```python
from build123d import *

# Parameters (mm, degrees)
SKETCH2_W           = 30.4
SKETCH2_H           = 30.4
BOSS_EXTRUDE1_DEPTH = 6
FILLET1_R           = 5
FILLET2_R           = 1
CUT_EXTRUDE1_DEPTH  = 0.5
BOSS_EXTRUDE2_DEPTH = 6.6
CUT_EXTRUDE2_DEPTH  = 10.6
FILLET3_R           = 1
CUT_EXTRUDE3_REACH  = 32.4
SKETCH9_W           = 0.8
SKETCH9_H           = 5.55
BOSS_EXTRUDE5_DEPTH = 2.35
LPATTERN1_COUNT     = 5
LPATTERN1_PITCH     = 2.78
SKETCH10_W          = 11.92
SKETCH10_H          = 2.35
BOSS_EXTRUDE6_DEPTH = 1
BOSS_EXTRUDE7_DEPTH = 1.65
SKETCH12_R          = 3.5
SKETCH12_R_2        = 2.5
BOSS_EXTRUDE8_DEPTH = 3.99
BOSS_EXTRUDE9_DEPTH = 1.6


with BuildPart() as part:
    # Sketch2 → Boss-Extrude1 (new body)
    with BuildSketch(Plane.XZ.offset(1.6)):
        with Locations((0, -13.5)):
            Rectangle(SKETCH2_W, SKETCH2_H)
    extrude(amount=BOSS_EXTRUDE1_DEPTH)

    # Fillet1
    fillet1_edges = [part.edges().sort_by_distance(p)[0] for p in [
        (15.2, -4.6, -28.7),
        (-15.2, -4.6, -28.7),
        (-15.2, -4.6, 1.7),
        (15.2, -4.6, 1.7),
    ]]
    fillet(fillet1_edges, radius=FILLET1_R)

    # Fillet2
    fillet2_edges = [part.edges().sort_by_distance(p)[0] for p in [
        (0, -7.6, 1.7),
        (15.2, -7.6, -13.5),
        (-15.2, -7.6, -13.5),
        (0, -7.6, -28.7),
        (-13.735533906, -7.6, -27.235533906),
        (-13.735533906, -7.6, 0.235533906),
        (13.735533906, -7.6, -27.235533906),
        (13.735533906, -7.6, 0.235533906),
    ]]
    fillet(fillet2_edges, radius=FILLET2_R)

    # Sketch3 → Cut-Extrude1 (cut)
    with BuildSketch(Plane.XZ.offset(7.6)):
        with BuildLine():
            Line((10.2, -1.8), (-10.2, -1.8))
            ThreePointArc((-10.2, -1.8), (-11.260660172, -2.239339828), (-11.7, -3.3))
            Line((-11.7, -3.3), (-11.7, -23.7))
            ThreePointArc((-11.7, -23.7), (-11.260660172, -24.760660172), (-10.2, -25.2))
            Line((-10.2, -25.2), (10.2, -25.2))
            ThreePointArc((10.2, -25.2), (11.260660172, -24.760660172), (11.7, -23.7))
            Line((11.7, -23.7), (11.7, -3.3))
            ThreePointArc((11.7, -3.3), (11.260660172, -2.239339828), (10.2, -1.8))
        make_face()
    extrude(amount=-CUT_EXTRUDE1_DEPTH, mode=Mode.SUBTRACT)

    # Sketch4 → Boss-Extrude2 (add)
    with BuildSketch(Plane(origin=(0, -1.6, 0), x_dir=(1, 0, 0), z_dir=(0, 1, 0))):
        with BuildLine():
            Line((15.2, 23.7), (15.2, 3.3))
            ThreePointArc((15.2, 3.3), (13.735533906, -0.235533906), (10.2, -1.7))
            Line((10.2, -1.7), (-10.2, -1.7))
            ThreePointArc((-10.2, -1.7), (-13.735533906, -0.235533906), (-15.2, 3.3))
            Line((-15.2, 3.3), (-15.2, 23.7))
            ThreePointArc((-15.2, 23.7), (-13.735533906, 27.235533906), (-10.2, 28.7))
            Line((-10.2, 28.7), (10.2, 28.7))
            ThreePointArc((10.2, 28.7), (13.735533906, 27.235533906), (15.2, 23.7))
        make_face()
    extrude(amount=BOSS_EXTRUDE2_DEPTH)

    # Sketch5 → Cut-Extrude2 (cut)
    with BuildSketch(Plane(origin=(0, 5, 0), x_dir=(1, 0, 0), z_dir=(0, 1, 0))):
        with BuildLine():
            Line((10.2, 27.2), (-10.2, 27.2))
            ThreePointArc((-10.2, 27.2), (-12.674873734, 26.174873734), (-13.7, 23.7))
            Line((-13.7, 23.7), (-13.7, 3.3))
            ThreePointArc((-13.7, 3.3), (-12.674873734, 0.825126266), (-10.2, -0.2))
            Line((-10.2, -0.2), (10.2, -0.2))
            ThreePointArc((10.2, -0.2), (12.674873734, 0.825126266), (13.7, 3.3))
            Line((13.7, 3.3), (13.7, 23.7))
            ThreePointArc((13.7, 23.7), (12.674873734, 26.174873734), (10.2, 27.2))
        make_face()
    extrude(amount=-CUT_EXTRUDE2_DEPTH, mode=Mode.SUBTRACT)

    # Fillet3
    fillet3_edges = [part.edges().sort_by_distance(p)[0] for p in [
        (13.735533906, 5, -27.235533906),
        (0, 5, -28.7),
        (-13.735533906, 5, -27.235533906),
        (-15.2, 5, -13.5),
        (-13.735533906, 5, 0.235533906),
        (0, 5, 1.7),
        (13.735533906, 5, 0.235533906),
        (15.2, 5, -13.5),
    ]]
    fillet(fillet3_edges, radius=FILLET3_R)

    # Sketch6 → Cut-Extrude3 (cut, up to next)
    with BuildSketch(Plane.XY.offset(1.7), mode=Mode.PRIVATE) as cut_extrude3_sk1:
        with BuildLine():
            Line((5.17, -2.55), (5.17, 5))
            Line((5.17, 5), (-5.17, 5))
            Line((-5.17, 5), (-5.17, -2.55))
            ThreePointArc((-5.17, -2.55), (-4.964974747, -3.044974747), (-4.47, -3.25))
            Line((-4.47, -3.25), (4.47, -3.25))
            ThreePointArc((4.47, -3.25), (4.964974747, -3.044974747), (5.17, -2.55))
        make_face()
    cut_extrude3_tool1 = extrude(cut_extrude3_sk1.sketch, amount=-CUT_EXTRUDE3_REACH, mode=Mode.PRIVATE) & part.part
    add(cut_extrude3_tool1.solids().sort_by_distance((0, 0.884808, 1.7))[0], mode=Mode.SUBTRACT)

    # Sketch9 → Boss-Extrude5 (add)
    with BuildSketch(Plane(origin=(0, -5.6, 0), x_dir=(1, 0, 0), z_dir=(0, 1, 0))):
        with Locations((5.57, 2.575)):
            Rectangle(SKETCH9_W, SKETCH9_H)
    boss_extrude5 = extrude(amount=BOSS_EXTRUDE5_DEPTH)

    # LPattern1: Boss-Extrude5 ×5
    with Locations(*[(-i * LPATTERN1_PITCH, 0, 0) for i in range(1, LPATTERN1_COUNT)]):
        add(boss_extrude5)

    # Sketch10 → Boss-Extrude6 (add)
    with BuildSketch(Plane(origin=(0, 0, -5.35), x_dir=(-1, 0, 0), z_dir=(0, 0, -1))):
        with Locations((-0.01, -4.425)):
            Rectangle(SKETCH10_W, SKETCH10_H)
    extrude(amount=-BOSS_EXTRUDE6_DEPTH)

    # Sketch11 → Boss-Extrude7 (add)
    with BuildSketch(Plane(origin=(0, -3.25, 0), x_dir=(1, 0, 0), z_dir=(0, 1, 0))):
        Polygon((-5.15, 4.35), (5.17, 4.35), (5.17, -0.2), (5.97, -0.2), (5.97, 5.35), (-5.95, 5.35), (-5.95, -0.2), (-5.15, -0.2), align=None)
    extrude(amount=BOSS_EXTRUDE7_DEPTH)

    # Sketch12 → Boss-Extrude8 (add)
    with BuildSketch(Plane(origin=(0, -5.6, 0), x_dir=(1, 0, 0), z_dir=(0, 1, 0))):
        with Locations((10, 3.5)):
            Circle(SKETCH12_R)
        with Locations((10, 3.5)):
            Circle(SKETCH12_R_2, mode=Mode.SUBTRACT)
        with Locations((10, 23.5)):
            Circle(SKETCH12_R)
        with Locations((10, 23.5)):
            Circle(SKETCH12_R_2, mode=Mode.SUBTRACT)
        with Locations((-10, 23.5)):
            Circle(SKETCH12_R)
        with Locations((-10, 23.5)):
            Circle(SKETCH12_R_2, mode=Mode.SUBTRACT)
        with Locations((-10, 3.5)):
            Circle(SKETCH12_R)
        with Locations((-10, 3.5)):
            Circle(SKETCH12_R_2, mode=Mode.SUBTRACT)
    extrude(amount=BOSS_EXTRUDE8_DEPTH)

    # Sketch13 → Boss-Extrude9 (add)
    with BuildSketch(Plane(origin=(0, -1.6, 0), x_dir=(1, 0, 0), z_dir=(0, 1, 0))):
        with BuildLine():
            Line((-5.95, -0.2), (-5.15, -0.2))
            Line((-5.15, -0.2), (-5.15, 4.33366661))
            ThreePointArc((-5.15, 4.33366661), (-5.67023311, 4.063914275), (-5.95, 3.548997487))
            Line((-5.95, 3.548997487), (-5.95, -0.2))
        make_face()
        with BuildLine():
            Line((5.17, -0.2), (5.97, -0.2))
            Line((5.97, -0.2), (5.97, 3.35))
            ThreePointArc((5.97, 3.35), (5.744596669, 3.982455532), (5.17, 4.329795897))
            Line((5.17, 4.329795897), (5.17, -0.2))
        make_face()
    extrude(amount=BOSS_EXTRUDE9_DEPTH)


solid = part.part
```
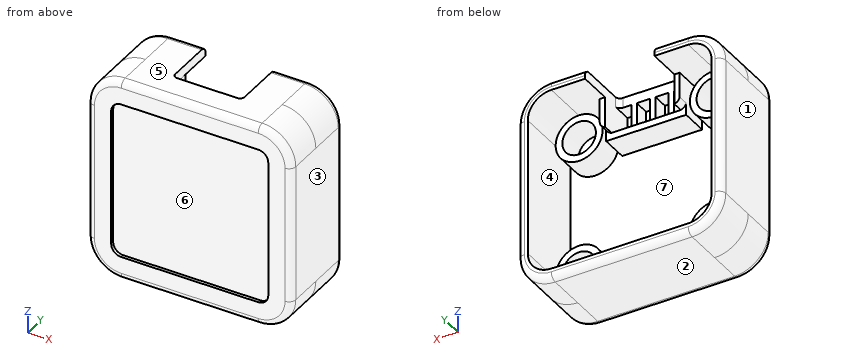
Source: CAD feature listing. Evaluate the final solid. Frame: model axes, mm. Face numbers are marked on the shaded views. A direction names the side the tool comes from. Round coordinates to 2 decimals unless told otherwise and drop trailing zeros. Write each loop counter-clockwise with the first axis right and the second up, starting at its lowest first coordinate (ties: lowest second). Pieces come first, ordered by that corner, then holes. Notation, with made-up numbers: M -33.5,-5.75 L 3.5,-5.75 A24 ccw 3.5,6.25 Z; hole C 34.5,2 d4. An arc over 180 degrees is marked long. Answer as a JSON object with one key per item and string values. Group by question number.
(1) Section query B-B on x = 0. Output: boundary loops of the cut face in (y, z).
(2) First-contact query: pin 1 (0.8 mm diameter, centred on y = 3, z = 1, fed in from +X); pin 2 (2 mm diameter, centred on x = -4, z = -5.5, fed in from -Y); pin 3 (1.6 mm diameter, centred on x = -1, z = -1, fed in from +Y). Flat tips, straight axial feed; report the tip coordinate or a pass-through.
(3) Section query D-D on y = -4. State how many separate pieces and enclosed holes the cut face has, then the cut area to 3 significant figures.
(4) Ray query, line 1 (Z direction, x = 10, y = -4.55); line 2 (X direction, y = 3.5, z = -13); line 3 (X direction, y = -4.6, z = -23.5). Return the intervals inside material, ascending. Write a range as [from, to].
(5) Section query C-C on z = -11. Output: boundary loops of the cut face in (x, y).
(6) Reachability of the marked faces 5, 6 and 7 from +Z, -Z, +X, -X, +Y, -Y: full face, straight path, thin tool, end or side. Return the list, or none.
(7) Mould query, pull axis X, two halves, no side actions, for the marked faces 1, 2, 3 and 4. Classes: +X half, -X half, draft (parallel to the pull), parting line (faces both ways), or undercut.
Computed values:
{
 "1": {"outline": "M -7.6,-27.7 A1 ccw -6.6,-28.7 L 4,-28.7 A1 ccw 5,-27.7 L 5,-27.2 L -5.6,-27.2 L -5.6,-5.35 L -1.6,-5.35 L -1.6,-4.35 L -3.25,-4.35 L -3.25,1.7 L -6.6,1.7 A1 ccw -7.6,0.7 L -7.6,-1.8 L -7.1,-1.8 L -7.1,-25.2 L -7.6,-25.2 Z"},
 "2": {"pin 1": "x = 13.33", "pin 2": "y = -7.1", "pin 3": "y = -3.25"},
 "3": {"separate pieces": "5", "enclosed holes": "9", "area": "268 mm^2"},
 "4": {"line 1": "[-28.7, -27.2], [-27, -26], [-21, -20], [-7, -6], [-1, 0], [0.2, 1.7]", "line 2": "[-15.2, -13.7], [13.7, 15.2]", "line 3": "[-15.2, -13.7], [-13.5, -12.5], [-7.5, -6.5], [6.5, 7.5], [12.5, 13.5], [13.7, 15.2]"},
 "5": {"outline": "M -15.2,-6.6 A1 ccw -14.2,-7.6 L -11.7,-7.6 L -11.7,-7.1 L 11.7,-7.1 L 11.7,-7.6 L 14.2,-7.6 A1 ccw 15.2,-6.6 L 15.2,4 A1 ccw 14.2,5 L 13.7,5 L 13.7,-5.6 L -13.7,-5.6 L -13.7,5 L -14.2,5 A1 ccw -15.2,4 Z"},
 "6": {"face 5": "+Z, +X, -X, +Y, -Y", "face 6": "-Y", "face 7": "+Y"},
 "7": {"face 1": "-X half", "face 2": "draft", "face 3": "+X half", "face 4": "undercut"}
}
